from build123d import *

# Parameters (mm, degrees)
CUT_EXTRUDE1_DEPTH = 5.582296376


with BuildPart() as part:
    # Sketch1 → Revolve2 (revolve)
    with BuildSketch(Plane.XY, mode=Mode.PRIVATE) as revolve2_sk:
        with BuildLine():
            Line((1.432534745, 7.84625121), (-0.067914271, 7.84625121))
            Line((-0.067914271, 7.84625121), (-0.067914271, 7.73195121))
            Line((-0.067914271, 7.73195121), (1.432534745, 7.73195121))
            ThreePointArc((1.432534745, 7.73195121), (1.534596416, 7.711649881), (1.621120123, 7.653836588))
            Line((1.621120123, 7.653836588), (1.90593549, 7.369021221))
            ThreePointArc((1.90593549, 7.369021221), (2.065565133, 7.255760643), (2.256165479, 7.21125121))
            Line((2.256165479, 7.21125121), (3.106859566, 7.21125121))
            Line((3.106859566, 7.21125121), (3.106859566, 7.33825121))
            Line((3.106859566, 7.33825121), (2.256165479, 7.33825121))
            ThreePointArc((2.256165479, 7.33825121), (2.110363091, 7.367253108), (1.986757795, 7.449843526))
            Line((1.986757795, 7.449843526), (1.701942428, 7.734658893))
            ThreePointArc((1.701942428, 7.734658893), (1.578337132, 7.817249312), (1.432534745, 7.84625121))
        make_face()
    revolve(revolve2_sk.sketch.rotate(Axis((-0.067914271, 7.84625121, 0), (0, -1, 0)), 90), axis=Axis((-0.067914271, 7.84625121, 0), (0, -1, 0)))

    # Sketch2 → Cut-Extrude1 (cut, through all)
    with BuildSketch(Plane.XZ.offset(-7.21125121)):
        with BuildLine():
            Line((2.090859566, -0.5715), (2.090859566, -0.6985))
            ThreePointArc((2.090859566, -0.6985), (2.165254443, -0.878105122), (2.344859566, -0.9525))
            Line((2.344859566, -0.9525), (3.634475543, -0.9525))
            Line((3.634475543, -0.9525), (3.634475543, -0.3175))
            Line((3.634475543, -0.3175), (2.344859566, -0.3175))
            ThreePointArc((2.344859566, -0.3175), (2.165254443, -0.391894878), (2.090859566, -0.5715))
        make_face()
        with BuildLine():
            Line((2.344859566, 0.9525), (3.634475543, 0.9525))
            Line((3.634475543, 0.9525), (3.634475543, 0.3175))
            Line((3.634475543, 0.3175), (2.344859566, 0.3175))
            ThreePointArc((2.344859566, 0.3175), (2.165254443, 0.391894878), (2.090859566, 0.5715))
            Line((2.090859566, 0.5715), (2.090859566, 0.6985))
            ThreePointArc((2.090859566, 0.6985), (2.165254443, 0.878105122), (2.344859566, 0.9525))
        make_face()
    extrude(amount=-CUT_EXTRUDE1_DEPTH, mode=Mode.SUBTRACT)


solid = part.part
Model file for the job. Use its own axes, mm. Coordinates: 2 decimals unless noted, no trailing zeros. Order: outer loops, then holes, each group sorted by start corner. A loop starts at its lowest first (then second) coordinate and runs counter-clockwise, first axis right, second up. Notation, with made-up numbers: (74, 3) -> (85, 3) arc R7 ccw to (85, 12) -> close; hole circle Ø2 at (40, 84.5). An arc over 180 degrees is marked (long way). Return JSON: item names as keys, results as strings. Group by question number.
Item 1: Saw through at A-A on z = 0. Write the cut outline in (x, y).
Item 2: Wall check: line 1 along X through (y, z) = (7.5, 0); line 2 along Z through (x, y) = (-0.75, 7.55); line 3 along X through (y, z) = (7.3, -1.25). Give the ranges that are in metal, low to high. Write a range as [from, to].
Item 3: Flat gauge pin, fed straight in: P1, Ø1.5, axis at x = 0, z = -1.5, coming from the -Y side. Where does the tip first touch, or does it go through?
Item 4: Saw through at B-B on z = 2.75. Write the cut outline in (x, y), then the cut area to 3 significant figures.
Values found:
{
 "1": {"outline": "(-3.24, 7.21) -> (-2.39, 7.21) arc R0.51 ccw to (-2.04, 7.37) -> (-1.76, 7.65) arc R0.27 cw to (-1.57, 7.73) -> (1.43, 7.73) arc R0.27 cw to (1.62, 7.65) -> (1.91, 7.37) arc R0.51 ccw to (2.26, 7.21) -> (3.11, 7.21) -> (3.11, 7.34) -> (2.26, 7.34) arc R0.38 cw to (1.99, 7.45) -> (1.7, 7.73) arc R0.38 ccw to (1.43, 7.85) -> (-1.57, 7.85) arc R0.38 ccw to (-1.84, 7.73) -> (-2.12, 7.45) arc R0.38 cw to (-2.39, 7.34) -> (-3.24, 7.34) -> close"},
 "2": {"line 1": "x = [-2.07, -1.91], [1.77, 1.94]", "line 2": "z = [-1.83, -1.66], [1.66, 1.83]", "line 3": "x = [-2.99, -1.7], [1.56, 2.85]"},
 "3": {"P1": "stops at y = 7.22"},
 "4": {"outline": "(-1.65, 7.21) -> (1.52, 7.21) -> (1.52, 7.34) -> (-1.65, 7.34) -> close", "area": "0.403 mm2"}
}
